For this review, take the finished solid that the model builds, in its own axes (mm). Round coordinates to 2 decimals unless told otherwise and drop trailing zeros. Loops run counter-clockwise (first coordinate to the right, second up) from the corner with the lowest first, then second, coordinate; pieces in that order, holes last.
1. Consider section A-A on x = -131. State the section outline as (y, z) points.
2. To check wall thickness, follow line 1 along Y through (x, z) = (-26, 0.25); line 2 along Y through (x, z) = (-282, 0.4); line 3 along Z through (x, y) = (-165, -0.75). State the ranges of each line that lie inside material, in increasing order.
3. Consider section B-B on y = 1.1. State the section outline as (x, z) points, then the cut area to 3 significant figures.
4. Consider section C-C on z = -1.35. State the section outline as (x, y) points.
5. Clearance check with a flat-ended pin moving along its axis: pin 1 Ø1 at (x, z) = (-178.5, -1.5) entering from +Y. State where the tip first meets the part, or that it passes through.
from build123d import *

# Parameters (mm, degrees)
F0_R     = 2.38125
F1_DEPTH = 482.6
F2_R     = 6.096
F2_R_2   = 1.5875
F3_DEPTH = 3.175


with BuildPart() as f1:
    # F0 (on Right) → F1 (new body)
    with BuildSketch(Plane.YZ):
        Circle(F0_R)
    extrude(amount=-F1_DEPTH)


with BuildPart() as f3:
    # F2 (on Right) → F3 (new body)
    with BuildSketch(Plane.YZ):
        with Locations((-50.084271, 0)):
            Circle(F2_R)
        with Locations((-50.084271, 0)):
            Circle(F2_R_2, mode=Mode.SUBTRACT)
    extrude(amount=-F3_DEPTH)


solid = f1.part
Resolved:
1. outline: circle Ø4.76 at (0, 0)
2. line 1: y = -2.37 to 2.37
2. line 2: y = -2.35 to 2.35
2. line 3: z = -2.26 to 2.26
3. outline: (-482.6, -2.11) - (0, -2.11) - (0, 2.11) - (-482.6, 2.11) - close
3. area: 2,040 mm2
4. outline: (-482.6, -1.96) - (0, -1.96) - (0, 1.96) - (-482.6, 1.96) - close
5. pin 1: stops at y = 2.16
